CAD build for the part. Positions are in the model's coordinates, mm. A direction names the side the tool comes from. Give positions to 0.01 mm unless a question says otherwise; leave off trailing zeros. Loops run counter-clockwise (first coordinate to the right, second up) from the corner with the lowest first, then second, coordinate; pieces in that order, holes last. Notation, with made-up numbers: M -5.75,44 L 23.25,44 A22 ccw 23.25,75 Z; hole C -21.5,-4.75 d9. An arc over 180 degrees is marked long. Answer as CSV lines item,"result".
from build123d import *

# Parameters (mm, degrees)
F1_DEPTH = 50.8
F2_DEPTH = 152.4
F3_DEPTH = 508
F4_W     = 495.3
F4_H     = 254
F4_W_2   = 190.5
F4_H_2   = 127
F4_W_3   = 285.75
F4_H_3   = 50.8
F5_DEPTH = 6.35
F6_DEPTH = 254
F4_W_4   = 12.7
F4_R     = 12.7
F7_DEPTH = 19.05


with BuildPart() as f1:
    # F0 (on Top) → F1 (new body)
    with BuildSketch(Plane.XY):
        with BuildLine():
            ThreePointArc((228.6, 123.825), (201.6592316368, 134.9842316368), (190.5, 161.925))
            Line((190.5, 161.925), (-190.5, 161.925))
            ThreePointArc((-190.5, 161.925), (-201.6592316368, 134.9842316368), (-228.6, 123.825))
            Line((-228.6, 123.825), (-228.6, -123.825))
            ThreePointArc((-228.6, -123.825), (-201.6592316368, -134.9842316368), (-190.5, -161.925))
            Line((-190.5, -161.925), (190.5, -161.925))
            ThreePointArc((190.5, -161.925), (201.6592316368, -134.9842316368), (228.6, -123.825))
            Line((228.6, -123.825), (228.6, 123.825))
        make_face()
        with BuildLine():
            ThreePointArc((-228.6, 123.825), (-201.6592316368, 134.9842316368), (-190.5, 161.925))
            Line((-190.5, 161.925), (-228.6, 161.925))
            Line((-228.6, 161.925), (-228.6, 123.825))
        make_face()
        with BuildLine():
            ThreePointArc((-190.5, -161.925), (-201.6592316368, -134.9842316368), (-228.6, -123.825))
            Line((-228.6, -123.825), (-228.6, -161.925))
            Line((-228.6, -161.925), (-190.5, -161.925))
        make_face()
        with BuildLine():
            Line((228.6, -161.925), (228.6, -123.825))
            ThreePointArc((228.6, -123.825), (201.6592316368, -134.9842316368), (190.5, -161.925))
            Line((190.5, -161.925), (228.6, -161.925))
        make_face()
        with BuildLine():
            Line((228.6, 161.925), (190.5, 161.925))
            ThreePointArc((190.5, 161.925), (201.6592316368, 134.9842316368), (228.6, 123.825))
            Line((228.6, 123.825), (228.6, 161.925))
        make_face()
    extrude(amount=-F1_DEPTH)

    # F0 (on Top) → F2 (join)
    with BuildSketch(Plane.XY):
        with BuildLine():
            ThreePointArc((-228.6, -123.825), (-255.5407683632, -134.9842316368), (-266.7, -161.925))
            ThreePointArc((-266.7, -161.925), (-255.540768159, -188.8657685674), (-228.5999994224, -200.025))
            ThreePointArc((-228.5999994224, -200.025), (-201.6592314326, -188.865768159), (-190.5, -161.925))
            Line((-190.5, -161.925), (-228.6, -161.925))
            Line((-228.6, -161.925), (-228.6, -123.825))
        make_face()
        with BuildLine():
            ThreePointArc((-190.5, -161.925), (-201.6592316368, -134.9842316368), (-228.6, -123.825))
            Line((-228.6, -123.825), (-228.6, -161.925))
            Line((-228.6, -161.925), (-190.5, -161.925))
        make_face()
        with BuildLine():
            ThreePointArc((-228.6, 123.825), (-201.6592316368, 134.9842316368), (-190.5, 161.925))
            Line((-190.5, 161.925), (-228.6, 161.925))
            Line((-228.6, 161.925), (-228.6, 123.825))
        make_face()
        with BuildLine():
            ThreePointArc((-190.5, 161.925), (-201.6592316368, 188.8657683632), (-228.6, 200.025))
            ThreePointArc((-228.6, 200.025), (-255.5407683632, 188.8657683632), (-266.7, 161.925))
            ThreePointArc((-266.7, 161.925), (-255.5407683632, 134.9842316368), (-228.6, 123.825))
            Line((-228.6, 123.825), (-228.6, 161.925))
            Line((-228.6, 161.925), (-190.5, 161.925))
        make_face()
        with BuildLine():
            Line((228.6, 161.925), (190.5, 161.925))
            ThreePointArc((190.5, 161.925), (201.6592316368, 134.9842316368), (228.6, 123.825))
            Line((228.6, 123.825), (228.6, 161.925))
        make_face()
        with BuildLine():
            ThreePointArc((266.7, 161.925), (255.5407683632, 188.8657683632), (228.6, 200.025))
            ThreePointArc((228.6, 200.025), (201.6592316368, 188.8657683632), (190.5, 161.925))
            Line((190.5, 161.925), (228.6, 161.925))
            Line((228.6, 161.925), (228.6, 123.825))
            ThreePointArc((228.6, 123.825), (255.5407683632, 134.9842316368), (266.7, 161.925))
        make_face()
        with BuildLine():
            Line((228.6, -161.925), (228.6, -123.825))
            ThreePointArc((228.6, -123.825), (201.6592316368, -134.9842316368), (190.5, -161.925))
            Line((190.5, -161.925), (228.6, -161.925))
        make_face()
        with BuildLine():
            ThreePointArc((228.6, -200.025), (255.5407683632, -188.8657683632), (266.7, -161.925))
            ThreePointArc((266.7, -161.925), (255.5407683632, -134.9842316368), (228.6, -123.825))
            Line((228.6, -123.825), (228.6, -161.925))
            Line((228.6, -161.925), (190.5, -161.925))
            ThreePointArc((190.5, -161.925), (201.6592316368, -188.8657683632), (228.6, -200.025))
        make_face()
    extrude(amount=-F2_DEPTH)

    # F0 (on Top) → F3 (join)
    with BuildSketch(Plane.XY):
        with BuildLine():
            ThreePointArc((-228.6, 123.825), (-255.5407683632, 134.9842316368), (-266.7, 161.925))
            Line((-266.7, 161.925), (-266.7, -161.925))
            ThreePointArc((-266.7, -161.925), (-255.5407683632, -134.9842316368), (-228.6, -123.825))
            Line((-228.6, -123.825), (-228.6, 123.825))
        make_face()
        with BuildLine():
            ThreePointArc((-266.7, 161.925), (-255.5407683632, 188.8657683632), (-228.6, 200.025))
            Line((-228.6, 200.025), (-266.7, 200.025))
            Line((-266.7, 200.025), (-266.7, 161.925))
        make_face()
        with BuildLine():
            ThreePointArc((-190.5, 161.925), (-201.6592316368, 188.8657683632), (-228.6, 200.025))
            ThreePointArc((-228.6, 200.025), (-255.5407683632, 188.8657683632), (-266.7, 161.925))
            ThreePointArc((-266.7, 161.925), (-255.5407683632, 134.9842316368), (-228.6, 123.825))
            Line((-228.6, 123.825), (-228.6, 161.925))
            Line((-228.6, 161.925), (-190.5, 161.925))
        make_face()
        with BuildLine():
            ThreePointArc((-228.6, 123.825), (-201.6592316368, 134.9842316368), (-190.5, 161.925))
            Line((-190.5, 161.925), (-228.6, 161.925))
            Line((-228.6, 161.925), (-228.6, 123.825))
        make_face()
        with BuildLine():
            ThreePointArc((228.6, 123.825), (201.6592316368, 134.9842316368), (190.5, 161.925))
            Line((190.5, 161.925), (-190.5, 161.925))
            ThreePointArc((-190.5, 161.925), (-201.6592316368, 134.9842316368), (-228.6, 123.825))
            Line((-228.6, 123.825), (-228.6, -123.825))
            ThreePointArc((-228.6, -123.825), (-201.6592316368, -134.9842316368), (-190.5, -161.925))
            Line((-190.5, -161.925), (190.5, -161.925))
            ThreePointArc((190.5, -161.925), (201.6592316368, -134.9842316368), (228.6, -123.825))
            Line((228.6, -123.825), (228.6, 123.825))
        make_face()
        with BuildLine():
            ThreePointArc((-190.5, -161.925), (-201.6592316368, -134.9842316368), (-228.6, -123.825))
            Line((-228.6, -123.825), (-228.6, -161.925))
            Line((-228.6, -161.925), (-190.5, -161.925))
        make_face()
        with BuildLine():
            ThreePointArc((-228.6, -123.825), (-255.5407683632, -134.9842316368), (-266.7, -161.925))
            ThreePointArc((-266.7, -161.925), (-255.540768159, -188.8657685674), (-228.5999994224, -200.025))
            ThreePointArc((-228.5999994224, -200.025), (-201.6592314326, -188.865768159), (-190.5, -161.925))
            Line((-190.5, -161.925), (-228.6, -161.925))
            Line((-228.6, -161.925), (-228.6, -123.825))
        make_face()
        with BuildLine():
            ThreePointArc((-228.5999994224, -200.025), (-255.540768159, -188.8657685674), (-266.7, -161.925))
            Line((-266.7, -161.925), (-266.7, -200.025))
            Line((-266.7, -200.025), (-228.5999994224, -200.025))
        make_face()
        with BuildLine():
            Line((-228.5999994224, -200.025), (228.6, -200.025))
            ThreePointArc((228.6, -200.025), (201.6592316368, -188.8657683632), (190.5, -161.925))
            Line((190.5, -161.925), (-190.5, -161.925))
            ThreePointArc((-190.5, -161.925), (-201.6592314326, -188.865768159), (-228.5999994224, -200.025))
        make_face()
        with BuildLine():
            ThreePointArc((228.6, -200.025), (255.5407683632, -188.8657683632), (266.7, -161.925))
            ThreePointArc((266.7, -161.925), (255.5407683632, -134.9842316368), (228.6, -123.825))
            Line((228.6, -123.825), (228.6, -161.925))
            Line((228.6, -161.925), (190.5, -161.925))
            ThreePointArc((190.5, -161.925), (201.6592316368, -188.8657683632), (228.6, -200.025))
        make_face()
        with BuildLine():
            Line((266.7, -200.025), (266.7, -161.925))
            ThreePointArc((266.7, -161.925), (255.5407683632, -188.8657683632), (228.6, -200.025))
            Line((228.6, -200.025), (266.7, -200.025))
        make_face()
        with BuildLine():
            Line((228.6, -161.925), (228.6, -123.825))
            ThreePointArc((228.6, -123.825), (201.6592316368, -134.9842316368), (190.5, -161.925))
            Line((190.5, -161.925), (228.6, -161.925))
        make_face()
        with BuildLine():
            Line((266.7, -161.925), (266.7, 161.925))
            ThreePointArc((266.7, 161.925), (255.5407683632, 134.9842316368), (228.6, 123.825))
            Line((228.6, 123.825), (228.6, -123.825))
            ThreePointArc((228.6, -123.825), (255.5407683632, -134.9842316368), (266.7, -161.925))
        make_face()
        with BuildLine():
            ThreePointArc((190.5, 161.925), (201.6592316368, 188.8657683632), (228.6, 200.025))
            Line((228.6, 200.025), (-228.6, 200.025))
            ThreePointArc((-228.6, 200.025), (-201.6592316368, 188.8657683632), (-190.5, 161.925))
            Line((-190.5, 161.925), (190.5, 161.925))
        make_face()
        with BuildLine():
            Line((266.7, 161.925), (266.7, 200.025))
            Line((266.7, 200.025), (228.6, 200.025))
            ThreePointArc((228.6, 200.025), (255.5407683632, 188.8657683632), (266.7, 161.925))
        make_face()
        with BuildLine():
            ThreePointArc((266.7, 161.925), (255.5407683632, 188.8657683632), (228.6, 200.025))
            ThreePointArc((228.6, 200.025), (201.6592316368, 188.8657683632), (190.5, 161.925))
            Line((190.5, 161.925), (228.6, 161.925))
            Line((228.6, 161.925), (228.6, 123.825))
            ThreePointArc((228.6, 123.825), (255.5407683632, 134.9842316368), (266.7, 161.925))
        make_face()
        with BuildLine():
            Line((228.6, 161.925), (190.5, 161.925))
            ThreePointArc((190.5, 161.925), (201.6592316368, 134.9842316368), (228.6, 123.825))
            Line((228.6, 123.825), (228.6, 161.925))
        make_face()
    extrude(amount=F3_DEPTH)

    # F4 (on face) → F5 (cut)
    with BuildSketch(Plane.XZ.offset(200.025)):
        Polygon((266.7, 508), (-266.7, 508), (-266.7, 0), (-228.6, 0), (228.6, 0), (266.7, 0), align=None)
        with Locations((0, 146.05)):
            Rectangle(F4_W, F4_H, mode=Mode.SUBTRACT)
        with Locations((-152.4, 355.6)):
            Rectangle(F4_W_2, F4_H_2, mode=Mode.SUBTRACT)
        with Locations((104.775, 355.6)):
            Rectangle(F4_W_3, F4_H_2, mode=Mode.SUBTRACT)
        with Locations((0, 463.55)):
            Rectangle(F4_W, F4_H_3, mode=Mode.SUBTRACT)
    extrude(amount=-F5_DEPTH, mode=Mode.SUBTRACT)

    # F4 (on face) → F6 (join)
    with BuildSketch(Plane.XZ.offset(200.025)):
        with Locations((0, 463.55)):
            Rectangle(F4_W, F4_H_3)
    extrude(amount=F6_DEPTH)

    # F4 (on face) → F7 (join)
    with BuildSketch(Plane.XZ.offset(200.025)):
        with Locations((-190.5, 146.05)):
            Rectangle(F4_W_4, F4_H_2)
        with Locations((-107.95, 355.6)):
            Circle(F4_R)
        with Locations((12.7, 355.6)):
            Circle(F4_R)
    extrude(amount=F7_DEPTH)


solid = f1.part
1) Drill centre lines: line 1 (Y direction, x = -213, z = 122.5) (3 decimals); line 2 (Z direction, x = -168.5, y = 163); line 3 (Z direction, x = -66, y = 74.5). Where is each one in solid material? Low to high. Write a range as from..to.
Answer below:
line 1,"y = -200.025..200.025"
line 2,"z = 0..508"
line 3,"z = -50.8..508"
2) Mould opens along Y. For faces 1 (the face through (-3, -454.025, 464)), 2 (the face through (4, 200.025, 250)), 3 (the face through (247, 2, 0)), 4 (the face through (-4, 6, 508)) say: +Y half, -Y half, draft (parallel to the pull), parting line (faces both ways), or undercut.
Answer below:
face 1,"-Y half"
face 2,"+Y half"
face 3,"undercut"
face 4,"draft"
3) Band-saw the part on C-C on y = 66. Give the cut face in (x, z).
Answer below:
outline,"M -266.7,0 L -228.6,0 L -228.6,-50.8 L 228.6,-50.8 L 228.6,0 L 266.7,0 L 266.7,508 L -266.7,508 Z"
4) Band-saw the part on A-A on z = 109. Give the cut face in (x, y) (3 decimals).
Answer below:
outline,"M -266.7,-193.675 L -247.65,-193.675 L -247.65,-200.025 L -196.85,-200.025 L -196.85,-219.075 L -184.15,-219.075 L -184.15,-200.025 L 247.65,-200.025 L 247.65,-193.675 L 266.7,-193.675 L 266.7,200.025 L -266.7,200.025 Z"
5) Band-saw the part on B-B on x = -15. Give the cut face in (y, z) (3 decimals), and give its area (3 significant figures).
Answer below:
outline,"M -454.025,438.15 L -193.675,438.15 L -193.675,419.1 L -200.025,419.1 L -200.025,292.1 L -193.675,292.1 L -193.675,273.05 L -200.025,273.05 L -200.025,19.05 L -193.675,19.05 L -193.675,0 L -161.925,0 L -161.925,-50.8 L 161.925,-50.8 L 161.925,0 L 200.025,0 L 200.025,508 L -193.675,508 L -193.675,488.95 L -454.025,488.95 Z"
area,"232,000 mm^2"
6) Flat gauge pins, fed straight in: pin 1 (14 mm diameter, centred on x = -188, y = -207.5, fed in from -Z); pin 2 (12 mm diameter, centred on x = -126, z = 130, fed in from -Y) (3 decimals); pin 3 (1.9 mm diameter, centred on y = -198, z = 196, fed in from -X). Where does each tip first touch, or does it go through?
Answer below:
pin 1,"stops at z = 82.55"
pin 2,"stops at y = -200.025"
pin 3,"stops at x = -247.65"
7) Which spindle directions (+Z, -Z, +X, -X, +Y, -Y) get a long thin tool onto all of the face, cutting with end or side? Do faces 5 (the face through (-262, -186, 0)), 6 (the face through (-228.6, 2, -25)), 7 (the face through (228.6, -2, -25)). Say none if no direction does.
Answer below:
face 5,"-Z, -X, -Y"
face 6,"-Z, -X"
face 7,"-Z, +X"
8) Band-saw the part on D-D on z = 355.6. Give the cut face in (x, y) (3 decimals), and give its area (3 significant figures).
Answer below:
outline,"M -266.7,-193.675 L -247.65,-193.675 L -247.65,-200.025 L -120.65,-200.025 L -120.65,-219.075 L -95.25,-219.075 L -95.25,-200.025 L -57.15,-200.025 L -57.15,-193.675 L -38.1,-193.675 L -38.1,-200.025 L 0,-200.025 L 0,-219.075 L 25.4,-219.075 L 25.4,-200.025 L 247.65,-200.025 L 247.65,-193.675 L 266.7,-193.675 L 266.7,200.025 L -266.7,200.025 Z"
area,"214,000 mm^2"
